Check sheet for the modelled part. Datum: model origin and axes. Units: mm. Face numbers are marked on the shaded views. A direction names the side the tool comes from. Round coordinates to 2 decimals unless told otherwise and drop trailing zeros. Write each loop counter-clockwise with the first axis right and the second up, starting at its lowest first coordinate (ties: lowest second). Pieces come first, ordered by that corner, then holes.
from build123d import *

# Parameters (mm, degrees)
F1_DEPTH = 12.7
F3_D     = 6.35
F3_DEPTH = 25.4
F3_TIP   = 1.9077324654


with BuildPart() as f1:
    # F0 (on Top) → F1 (new body)
    with BuildSketch(Plane.XY):
        Polygon((39.4914927714, -23.0438545598), (39.4914927714, 0.2341428303), (36.910995181, 0.2341428303), (36.910995181, 23.1056753299), (24.210995181, 23.1056753299), (24.210995181, 0), (21.6304975905, 0), (21.6304975905, 23.1056753299), (8.9304975905, 23.1056753299), (8.9304975905, 0), (6.35, 0), (6.35, 23.1056753299), (0, 23.1056753299), (-6.35, 23.1056753299), (-6.35, 0), (-8.9304975905, 0), (-8.9304975905, 23.1056753299), (-21.6304975905, 23.1056753299), (-21.6304975905, 0), (-24.210995181, 0), (-24.210995181, 23.1056753299), (-36.910995181, 23.1056753299), (-36.910995181, 0.2341428303), (-39.4914927714, 0.2341428303), (-39.4914927714, -23.0438545598), (0, -23.0438545598), align=None)
    extrude(amount=F1_DEPTH)

    # F3
    with Locations(Plane(origin=(0, 23.1056753299, 0), x_dir=(-1, 0, 0), z_dir=(0, 1, 0))):
        with Locations((-30.560995181, 6.35)):
            Hole(F3_D / 2, depth=F3_DEPTH)
            with Locations((0, 0, -(F3_DEPTH + F3_TIP / 2))):  # 118° drill point
                Cone(0, F3_D / 2, F3_TIP, mode=Mode.SUBTRACT)


solid = f1.part
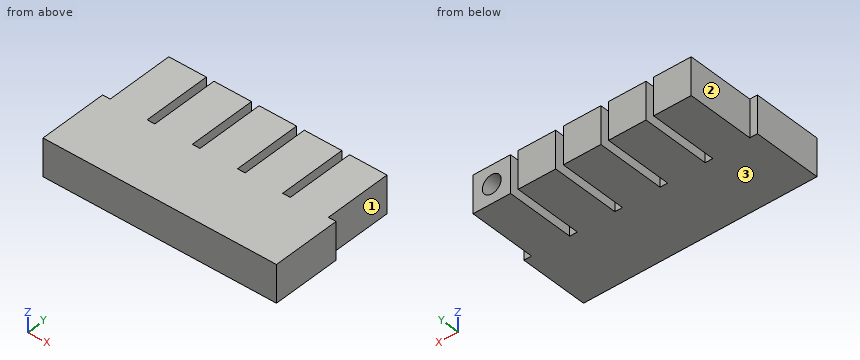
1. Sectioned sample at A-A, the plane y = 12.5. Give the number of separate pieces and of enclosed holes in the cut face, plus the area to 3 significant figures.
2. Set-up check for the marked faces 1, 2 and 3: record each of +Z, -Z, +X, -X, +Y, -Y from which the full face is reachable in a straight line by a thin tool's end or side.
3. Scan lines: line 1 along X through (y, z) = (5.5, 6.35); line 2 along X through (y, z) = (9, 11.75); line 3 along X through (y, z) = (6, 5). Record each from-to range of solid material in increasing order.
4. Sectioned sample at C-C, the plane x = 8. Enter the section's corners in (y, z), plus the area to 3 significant figures.
5. Sectioned sample at B-B, the plane z = 10.75. Enter the section's corners in (x, y), plus the area to 3 significant figures.
6. Go/stop test with flat-tipped pins: pin 1 (4 mm diameter, centred on y = 10.5, z = 9, fed in from -X); pin 2 (1 mm diameter, centred on x = -18.5, y = -3, fed in from -Z); pin 3 (0.8 mm diameter, centred on x = 8, z = 7.5, fed in from +Y); pin 4 (2 mm diameter, centred on x = 38.5, z = 4.5, fed in from +Y). Record where each tip stops, or that it passes through.
Computed values:
1. separate pieces: 5
1. enclosed holes: 1
1. area: 775 mm2
2. face 1: +Z, -Z, +X, +Y
2. face 2: +Z, -Z, -X, +Y
2. face 3: -Z, +X, -X, +Y, -Y
3. line 1: x = -36.91 to -24.21, -21.63 to -8.93, -6.35 to 6.35, 8.93 to 21.63, 24.21 to 27.39, 33.74 to 36.91
3. line 2: x = -36.91 to -24.21, -21.63 to -8.93, -6.35 to 6.35, 8.93 to 21.63, 24.21 to 36.91
3. line 3: x = -36.91 to -24.21, -21.63 to -8.93, -6.35 to 6.35, 8.93 to 21.63, 24.21 to 27.69, 33.43 to 36.91
4. outline: (-23.04, 0) - (0, 0) - (0, 12.7) - (-23.04, 12.7) - close
4. area: 293 mm2
5. outline: (-39.49, -23.04) - (39.49, -23.04) - (39.49, 0.23) - (36.91, 0.23) - (36.91, 23.11) - (24.21, 23.11) - (24.21, 0) - (21.63, 0) - (21.63, 23.11) - (8.93, 23.11) - (8.93, 0) - (6.35, 0) - (6.35, 23.11) - (-6.35, 23.11) - (-6.35, 0) - (-8.93, 0) - (-8.93, 23.11) - (-21.63, 23.11) - (-21.63, 0) - (-24.21, 0) - (-24.21, 23.11) - (-36.91, 23.11) - (-36.91, 0.23) - (-39.49, 0.23) - close
5. area: 3,290 mm2
6. pin 1: stops at x = -36.91
6. pin 2: stops at z = 0
6. pin 3: stops at y = 0
6. pin 4: stops at y = 0.23
